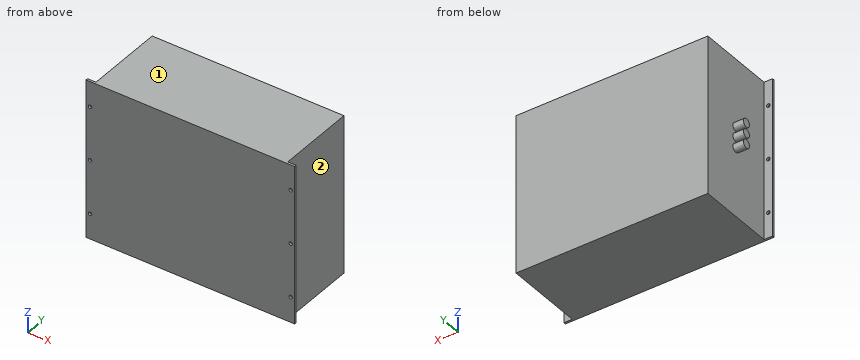
from build123d import *

# Parameters (mm, degrees)
SKETCH_1_W          = 182
SKETCH_1_H          = 150
EXTRUDE_1_DEPTH     = 77
SKETCH_2_W          = 8
SKETCH_2_H          = 150
EXTRUDE_2_DEPTH     = 2
SKETCH_3_R          = 1.7
CUT_EXTRUDE_1_DEPTH = 146.089627472
SKETCH_4_R          = 4
EXTRUDE_3_DEPTH     = 10


with BuildPart() as part:
    # 草图1 → 凸台-拉伸1 (new body)
    with BuildSketch(Plane(origin=(0, 0, 0), x_dir=(1, 0, 0), z_dir=(0, 1, 0))):
        Rectangle(SKETCH_1_W, SKETCH_1_H)
    extrude(amount=EXTRUDE_1_DEPTH)

    # 草图2 → 凸台-拉伸2 (add)
    with BuildSketch(Plane.XZ):
        with Locations((-95, 0)):
            Rectangle(SKETCH_2_W, SKETCH_2_H)
    extrude_2 = extrude(amount=-EXTRUDE_2_DEPTH)

    # 草图3 → 切除-拉伸1 (cut, through all)
    with BuildSketch(Plane(origin=(0, 2, 0), x_dir=(1, 0, 0), z_dir=(0, 1, 0))):
        with Locations(Location((-95.2, 51, 0), (0, 0, 270))):
            Circle(SKETCH_3_R)
        with Locations(Location((-95.2, -51, 0), (0, 0, 90))):
            Circle(SKETCH_3_R)
        with Locations(Location((-95.2, 0, 0), (0, 0, 270))):
            Circle(SKETCH_3_R)
    cut_extrude_1 = extrude(amount=-CUT_EXTRUDE_1_DEPTH, mode=Mode.SUBTRACT)

    # 镜向1: 凸台-拉伸2, 切除-拉伸1 across plane
    add(extrude_2.mirror(Plane(origin=(0, 0, 0), x_dir=(0, 0, 1), z_dir=(1, 0, 0))))
    add(cut_extrude_1.mirror(Plane(origin=(0, 0, 0), x_dir=(0, 0, 1), z_dir=(1, 0, 0))), mode=Mode.SUBTRACT)

    # 草图4 → 凸台-拉伸3 (add)
    with BuildSketch(Plane.ZY.offset(91)):
        with Locations(Location((0, 39.5, 0), (0, 0, 180))):
            Circle(SKETCH_4_R)
        with Locations(Location((10, 39.5, 0), (0, 0, 180))):
            Circle(SKETCH_4_R)
        with Locations(Location((-10, 39.5, 0), (0, 0, 180))):
            Circle(SKETCH_4_R)
    extrude(amount=EXTRUDE_3_DEPTH)


solid = part.part
Design review of the part built by this model. Coordinates are the model's own, in mm. Face numbers are marked on the shaded views. A direction names the side the tool comes from. Give positions to 0.01 mm unless a question says otherwise; leave off trailing zeros. Order: outer loops, then holes, each group sorted by start corner. A loop starts at its lowest first (then second) coordinate and runs counter-clockwise, first axis right, second up. Notation, with made-up numbers: (66.25, 32) - (84.25, 32) arc R18 ccw to (84.25, 60) - close; hole circle Ø5 at (73.25, 5.25). An arc over 180 degrees is marked (long way). Write item = value, one per line. Start each with the question number.
Q1. We need section B-B on y = 54.5. State the section outline as (x, z) points.
Q2. Clearance check with flat-ended pins moving along their axes: pin 1 Ø4.5 at (x, z) = (-95.2, -51) entering from +Y; pin 2 Ø4 at (y, z) = (57.5, 6.5) entering from -X; pin 3 Ø4 at (x, z) = (-95.2, 0) entering from +Y; pin 4 Ø3 at (x, z) = (95.2, 51) entering from +Y. State where each tip first meets the part, or that it passes through.
Q3. We need section A-A on z = 10. State the section outline as (x, y) points, plus the area to 3 significant figures.
Q4. We need section C-C on z = 61.5. State the section outline as (x, y) points.
Q5. To check wall thickness, follow L1, parallel to Z at x = 95, y = 1; L2, parallel to X at y = 1, z = 0; L3, parallel to X at y = 59, z = -13.5. State the ranges of each line that lie inside material, in increasing order. Write a range as from..to.
Q6. Tool access review of the marked faces 1 and 2: name each direction out of +Z, -Z, +X, -X, +Y, -Y from which nothing blocks a thin tool from reaching the whole face with its end or side.
Working result:
q1.outline = (-91, -75) - (91, -75) - (91, 75) - (-91, 75) - close
q2.pin_1 = 2
q2.pin_2 = -91
q2.pin_3 = 43.5
q2.pin_4 = through
q3.outline = (-101, 35.5) - (-91, 35.5) - (-91, 2) - (-99, 2) - (-99, 0) - (99, 0) - (99, 2) - (91, 2) - (91, 77) - (-91, 77) - (-91, 43.5) - (-101, 43.5) - close
q3.area = 14,100 mm²
q4.outline = (-99, 0) - (99, 0) - (99, 2) - (91, 2) - (91, 77) - (-91, 77) - (-91, 2) - (-99, 2) - close
q5.L1 = -75..-52.69, -49.31..-1.69, 1.69..49.31, 52.69..75
q5.L2 = -99..-96.9, -93.5..93.5, 96.9..99
q5.L3 = -91..91
q6.face_1 = +Z, +X, -X, +Y, -Y
q6.face_2 = +Z, -Z, +X, +Y
